CAD build for the part. Positions are in the model's coordinates, mm. A direction names the side the tool comes from. Coordinates: 2 decimals unless noted, no trailing zeros. Write each loop counter-clockwise with the first axis right and the second up, starting at its lowest first coordinate (ties: lowest second). Pieces come first, ordered by that corner, then holes. Notation, with made-up numbers: (45, -20.75) - (84, -20.75) arc R15 cw to (84, -10.75) - close; hole circle Ø4 at (19, 24.25). An arc over 180 degrees is marked (long way). One line per question, with ' | ' between items. Start each with the question number.
1. Band-saw the part on A-A, the plane y = -6.35. Write the cut outline in (x, z) (3 decimals), then the cut area to 3 significant figures.
2. Band-saw the part on D-D, the plane z = 14. Write the cut outline in (x, y).
3. Band-saw the part on B-B, the plane z = 81.5. Write the cut outline in (x, y), then the cut area to 3 significant figures.
4. Probe line 1 (Y direction, x = 0, z = 1.6) (3 decimals); line 2 (Y direction, x = -10.25, z = 81.5); line 3 (Z direction, x = -11, y = 29.5). List the from-to ranges inside material, lowest first.
5. Which spindle directions (+Z, -Z, +X, -X, +Y, -Y) get a long thin tool onto all of the face, cutting with end or side? Do faces 4 (the flat face through (-7.94, 1, 44)), 5 (the cylindrical face through (-0.36, -35.35, 1.08)). Say none if no direction does.
6. Band-saw the part on C-C, the plane y = -29.5. Write the cut outline in (x, z).
7. Two-plate mould, pull along Z, no slides. Class faces 1 (the flat face through (-9, -44.45, 39)), 2 (the flat face through (0, 1, 2.2)), 3 (the cylindrical face through (-10.9, 28.31, 5.28)): +Z half, -Z half, draft (parallel to the pull), parting line (faces both ways), or undercut.
8. Flat gauge pins, fed straight in: P1, Ø1.5, axis at y = -29.5, z = 81.5, coming from the -X side; P2, Ø1, axis at x = 5, y = -13, coming from the +Z side; P3, Ø12, axis at y = 21, z = 18, coming from the +X side. Where does each tip first touch, or does it go through?
from build123d import *

# Parameters (mm, degrees)
SKETCH_W     = 15.88
SKETCH_H     = 88.9
SKETCH_R     = 2.775
PAD_DEPTH    = 2.2
SKETCH001_W  = 88.9
SKETCH001_H  = 85
SKETCH001_R  = 1.25
PAD001_DEPTH = 6


with BuildPart() as part:
    # Sketch → Pad (new body)
    with BuildSketch(Plane.XY):
        Rectangle(SKETCH_W, SKETCH_H)
        with Locations((-0.0025, 38.1)):
            Circle(SKETCH_R, mode=Mode.SUBTRACT)
        with Locations((-0.0025, -38.1)):
            Circle(SKETCH_R, mode=Mode.SUBTRACT)
        with Locations((0, -6.35)):
            Circle(SKETCH_R, mode=Mode.SUBTRACT)
        with Locations((0, 6.35)):
            Circle(SKETCH_R, mode=Mode.SUBTRACT)
    extrude(amount=PAD_DEPTH)

    # Sketch001 (on Face4 of Pad) → Pad001 (join)
    with BuildSketch(Plane(origin=(-7.94, 0, 0), x_dir=(0, -1, 0), z_dir=(-1, 0, 0))):
        with Locations((0, 42.5)):
            Rectangle(SKETCH001_W, SKETCH001_H)
        with Locations((-29.5, 4.9)):
            Circle(SKETCH001_R, mode=Mode.SUBTRACT)
        with Locations((29.5, 4.9)):
            Circle(SKETCH001_R, mode=Mode.SUBTRACT)
        with Locations((29.5, 81.5)):
            Circle(SKETCH001_R, mode=Mode.SUBTRACT)
        with Locations((-29.5, 81.5)):
            Circle(SKETCH001_R, mode=Mode.SUBTRACT)
    extrude(amount=PAD001_DEPTH)


solid = part.part
Filled in:
1) outline: (-13.94, 0) - (-2.775, 0) - (-2.775, 2.2) - (-7.94, 2.2) - (-7.94, 85) - (-13.94, 85) - close; (2.775, 0) - (7.94, 0) - (7.94, 2.2) - (2.775, 2.2) - close | area: 533 mm²
2) outline: (-13.94, -44.45) - (-7.94, -44.45) - (-7.94, 44.45) - (-13.94, 44.45) - close
3) outline: (-13.94, -44.45) - (-7.94, -44.45) - (-7.94, -30.75) - (-13.94, -30.75) - close; (-13.94, -28.25) - (-7.94, -28.25) - (-7.94, 28.25) - (-13.94, 28.25) - close; (-13.94, 30.75) - (-7.94, 30.75) - (-7.94, 44.45) - (-13.94, 44.45) - close | area: 503 mm²
4) line 1: y = -44.45 to -40.875, -35.325 to -9.125, -3.575 to 3.575, 9.125 to 35.325, 40.875 to 44.45 | line 2: y = -44.45 to -30.75, -28.25 to 28.25, 30.75 to 44.45 | line 3: z = 0 to 3.65, 6.15 to 80.25, 82.75 to 85
5) face 4: +Z, +X, +Y, -Y | face 5: +Z, -Z
6) outline: (-13.94, 0) - (7.94, 0) - (7.94, 2.2) - (-7.94, 2.2) - (-7.94, 3.65) - (-13.94, 3.65) - close; (-13.94, 6.15) - (-7.94, 6.15) - (-7.94, 80.25) - (-13.94, 80.25) - close; (-13.94, 82.75) - (-7.94, 82.75) - (-7.94, 85) - (-13.94, 85) - close
7) face 1: draft | face 2: +Z half | face 3: undercut
8) P1: passes through | P2: stops at z = 2.2 | P3: stops at x = -7.94
